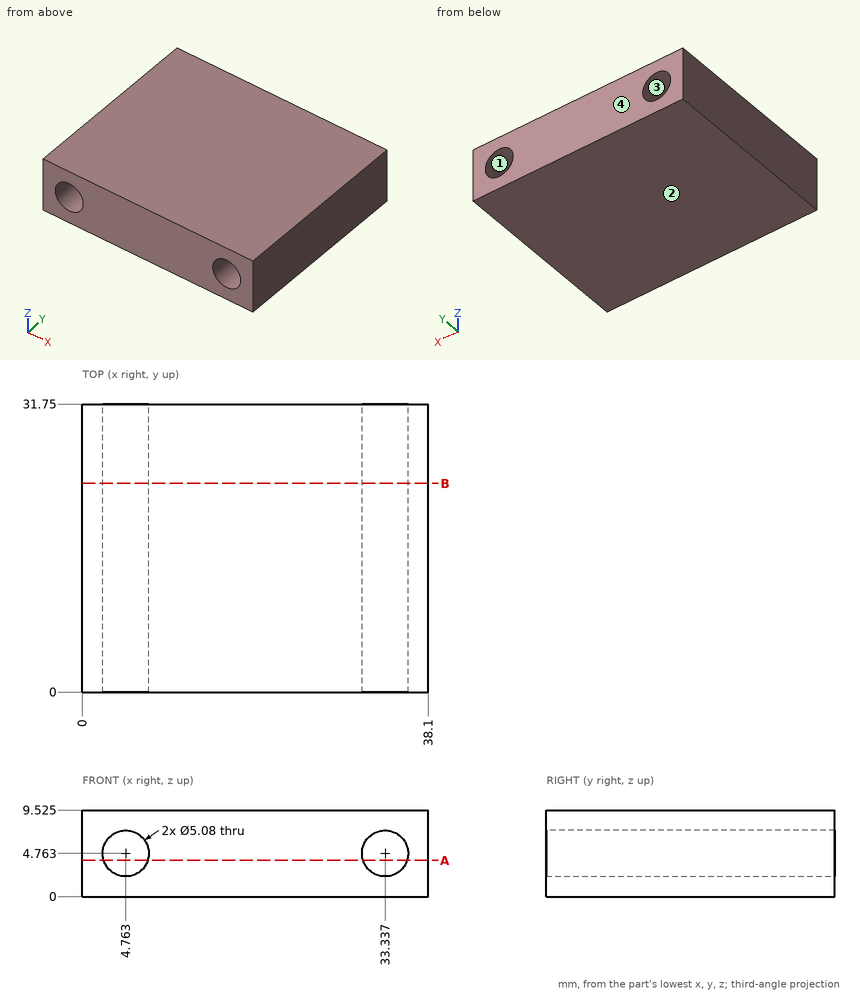
Study the drawing (mm; zero at the part's minimum x, y, z) and answer. Coordinates: 2 decimals unless noted, no trailing zeros. Loops run counter-clockwise (first coordinate to the right, second up) from the corner with the lowest first, then second, coordinate; pieces in that order, holes last. Notation, with made-up numbers: M 43.25,67.5 L 53.25,67.5 A19 cw 53.25,79.5 Z; hole C 16.5,-9.75 d9. An arc over 180 degrees is marked long. Answer in a Markdown table with one row per item.
1) Find the intervals of material crossed by probe 1 along X at (y, z) = (27, 4.75); probe 2 along X at (y, z) = (10, 7) (1 decimal); probe 3 along Z at (x, y) = (35, 26.5) (1 decimal), in increasing order.
Answers below:
| item | result |
|---|---|
| probe 1 | 0 to 2.22, 7.3 to 30.8, 35.88 to 38.1 |
| probe 2 | 0 to 3.6, 6 to 32.1, 34.5 to 38.1 |
| probe 3 | 0 to 2.8, 6.7 to 9.5 |
2) Determine the mould class of the marked faces 1, 2, 3 and 4 for opening direction Z: released by +Z, released by -Z, zero draft, split by the parting line, or undercut.
Answers below:
| item | result |
|---|---|
| face 1 | undercut |
| face 2 | released by -Z |
| face 3 | undercut |
| face 4 | zero draft |
3) Find section A-A (z = 4). Count the separate pieces of the cut face and the enclosed holes in it, then the cut area to 3 significant figures.
Answers below:
| item | result |
|---|---|
| separate pieces | 3 |
| enclosed holes | 0 |
| area | 902 mm^2 |
4) Find section B-B (y = 23). Determine the outline of the cut face in (x, z) (1 decimal), then the cut area to 3 significant figures.
Answers below:
| item | result |
|---|---|
| outline | M 0,0 L 38.1,0 L 38.1,9.5 L 0,9.5 Z; hole C 4.8,4.8 d5.1; hole C 33.3,4.8 d5.1 |
| area | 322 mm^2 |
5) Given pin 1 (4.5 mm diameter, centred on x = 33.34, z = 4.76, fed in from +Y), flat-ended and moving along its own axis, determine where the tip first touches the part or whether it passes through.
Answers below:
| item | result |
|---|---|
| pin 1 | through |
